Design review of the part built by this model. Coordinates are the model's own, in mm. A direction names the side the tool comes from. Round coordinates to 2 decimals unless told otherwise and drop trailing zeros. Write each loop counter-clockwise with the first axis right and the second up, starting at its lowest first coordinate (ties: lowest second). Pieces come first, ordered by that corner, then holes. Notation, with made-up numbers: M 47.25,-15.5 L 77.25,-15.5 A18 ccw 77.25,8.5 Z; hole C -18,55.25 d1. An arc over 180 degrees is marked long. One line per question, with ' | ' between items. Start each with the question number.
Item 1: Draft analysis for pull direction Y (two halves, no side actions). For faces 6 (the face through (90, 162, 6)), 7 (the face through (35, 160, 6)), 8 (the face through (79, 0, 6)), 9 (the face through (145, 15, 7)), state which applies: released by +Y, released by -Y, zero draft, split by the parting line, or undercut.
Item 2: Add section D-D, the plane x = 137. State the section outline as (y, z) points, and give its area (3 significant figures).
Item 3: Add section C-C, the plane x = 8.5. State the section outline as (y, z) points.
Item 4: For L1, parallel to X at y = 133.3, z = 4.5; L2, parallel to X at y = 133.3, z = 10.25; L3, parallel to Y at x = 8.5, z = 10.65, list the stretches that pass through material, from the lowest coordinate up.
Item 5: Insertion check: pin 1 Ø6 at (x, y) = (144, 19) entering from +Z; pin 2 Ø4.5 at (x, y) = (8.5, 133.3) entering from -Z; pin 3 Ø4.5 at (x, z) = (2.5, 6) entering from +Y. Each pin has a flat end and moves straight along its axis. Give the tip position at first contact, or say it passes through.
Item 6: Add section B-B, the plane z = 10. State the section outline as (x, y) points, and give its area (3 significant figures).
Item 7: Machinability: for faces 1 (the face through (2, 90.3, 6)), 2 (the face through (9.248, 129.932, 3.944)), 3 (the face through (81, 83, 0)), 4 (the face through (145, 4.75, 10)), 5 (the face through (162, 90, 6)), which of the approach directions +Z, -Z, +X, -X, +Y, -Y give a long, thin tool a straight path to every point of the face, cutting with its end or side? Answer none if there is none.
Item 8: Add section A-A, the plane y = 133.3. State the section outline as (x, z) points.
```python
from build123d import *

# Parameters (mm, degrees)
SKETCH1_R           = 2
BOSS_EXTRUDE1_DEPTH = 12
SKETCH2_W           = 20.5
SKETCH2_H           = 20.5
CUT_EXTRUDE1_DEPTH  = 5
SKETCH3_R           = 3.45
CUT_EXTRUDE2_DEPTH  = 8


with BuildPart() as part:
    # Sketch1 → Boss-Extrude1 (new body)
    with BuildSketch(Plane.XY):
        Polygon((0, 0), (69.7, 0), (90.3, 0), (160, 0), (160, 70), (164, 70), (164, 90), (160, 90), (160, 160), (90, 160), (90, 164), (70, 164), (70, 160), (0, 160), (0, 90.3), (4.2, 90.3), (4.2, 69.7), (0, 69.7), align=None)
        with Locations((8.5, 133.3)):
            Circle(SKETCH1_R, mode=Mode.SUBTRACT)
    extrude(amount=BOSS_EXTRUDE1_DEPTH)

    # Sketch2 → Cut-Extrude1 (cut)
    with BuildSketch(Plane.XY.offset(12)):
        with Locations((145, 15)):
            Rectangle(SKETCH2_W, SKETCH2_H)
    extrude(amount=-CUT_EXTRUDE1_DEPTH, mode=Mode.SUBTRACT)

    # Sketch3 → Cut-Extrude2 (cut)
    with BuildSketch(Plane(origin=(0, 0, 0), x_dir=(-1, 0, 0), z_dir=(0, 0, -1))):
        with Locations((-8.5, 133.3)):
            Circle(SKETCH3_R)
    extrude(amount=-CUT_EXTRUDE2_DEPTH, mode=Mode.SUBTRACT)


solid = part.part
```
Computed values:
1) face 6: zero draft | face 7: released by +Y | face 8: released by -Y | face 9: undercut
2) outline: M 0,0 L 160,0 L 160,12 L 25.25,12 L 25.25,7 L 4.75,7 L 4.75,12 L 0,12 Z | area: 1,820 mm^2
3) outline: M 0,0 L 129.85,0 L 129.85,8 L 131.3,8 L 131.3,12 L 0,12 Z; M 135.3,8 L 136.75,8 L 136.75,0 L 160,0 L 160,12 L 135.3,12 Z
4) L1: x = 0 to 5.05, 11.95 to 160 | L2: x = 0 to 6.5, 10.5 to 160 | L3: y = 0 to 131.3, 135.3 to 160
5) pin 1: stops at z = 7 | pin 2: stops at z = 8 | pin 3: stops at y = 160
6) outline: M 0,0 L 160,0 L 160,70 L 164,70 L 164,90 L 160,90 L 160,160 L 90,160 L 90,164 L 70,164 L 70,160 L 0,160 L 0,90.3 L 4.2,90.3 L 4.2,69.7 L 0,69.7 Z; hole C 8.5,133.3 d4; hole M 134.75,4.75 L 155.25,4.75 L 155.25,25.25 L 134.75,25.25 Z | area: 25,200 mm^2
7) face 1: +Z, -Z, -X | face 2: -Z | face 3: -Z, +X, -X, +Y, -Y | face 4: +Z | face 5: +Z, -Z, +X, +Y
8) outline: M 0,0 L 5.05,0 L 5.05,8 L 6.5,8 L 6.5,12 L 0,12 Z; M 10.5,8 L 11.95,8 L 11.95,0 L 160,0 L 160,12 L 10.5,12 Z
